Build history of the part. All positions in model axes, mm. Round coordinates to 2 decimals unless told otherwise and drop trailing zeros. Loops run counter-clockwise (first coordinate to the right, second up) from the corner with the lowest first, then second, coordinate; pieces in that order, holes last. Notation, with made-up numbers: (12.5, 33) - (49.5, 33) arc R18 cw to (49.5, 45) - close; hole circle Ø11 at (69.25, 8.5). An arc over 180 degrees is marked (long way). Put each result on its own line as item: value. Start each with the question number.
from build123d import *

# Parameters (mm, degrees)
BOSS_EXTRUDE1_DEPTH                             = 950
CBORE_FOR_M5_SOCKET_HEAD_CAP_SCREW2_D           = 5.5
CBORE_FOR_M5_SOCKET_HEAD_CAP_SCREW2_CBORE_D     = 10
CBORE_FOR_M5_SOCKET_HEAD_CAP_SCREW2_CBORE_DEPTH = 5
LPATTERN1_COUNT                                 = 16
LPATTERN1_PITCH                                 = 60


with BuildPart() as part:
    # Sketch1 → Boss-Extrude1 (new body)
    with BuildSketch(Plane.XY):
        Polygon((0, -9.237604307), (8, -4.618802154), (8, 4.618802154), (0, 9.237604307), (-8, 4.618802154), (-8, -4.618802154), align=None)
    extrude(amount=BOSS_EXTRUDE1_DEPTH)

    # CBORE for M5 Socket Head Cap Screw2 (through all)
    with Locations(Plane(origin=(8, 0, 925), x_dir=(0, 1, 0), z_dir=(1, 0, 0))):
        with Locations((0, 0)):
            cbore_for_m5_socket_head_cap_screw2 = CounterBoreHole(CBORE_FOR_M5_SOCKET_HEAD_CAP_SCREW2_D / 2, CBORE_FOR_M5_SOCKET_HEAD_CAP_SCREW2_CBORE_D / 2, CBORE_FOR_M5_SOCKET_HEAD_CAP_SCREW2_CBORE_DEPTH)

    # LPattern1: CBORE for M5 Socket Head Cap Screw2 ×16
    with Locations(*[(0, 0, -i * LPATTERN1_PITCH) for i in range(1, LPATTERN1_COUNT)]):
        add(cbore_for_m5_socket_head_cap_screw2, mode=Mode.SUBTRACT)


solid = part.part
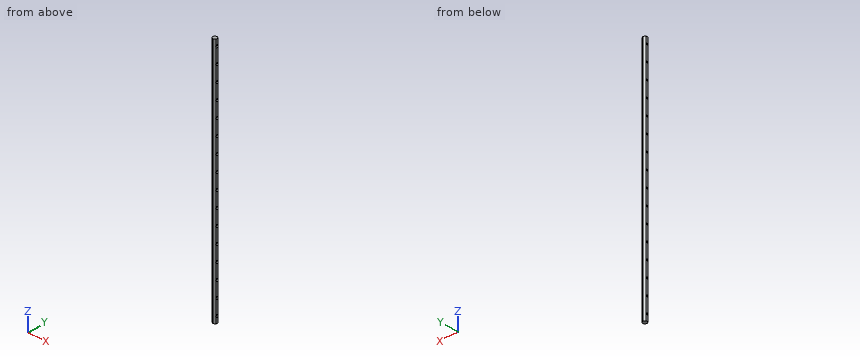
1) Slice it at A-A, the plane z = 541. Write the cut outline in (x, y), and give its area (3 significant figures).
2) Drill centre lines: line 1 (Y direction, x = -3, z = 625); line 2 (Y direction, x = 2.25, z = 209); line 3 (X direction, y = 6.25, z = 881). Where is each one in solid material? Low to high. Write a range as [from, to].
3) Drop flat-ended pins along their axis: pin 1 Ø9 at (y, z) = (0, 865) entering from +X; pin 2 Ø1 at (y, z) = (7, 113) entering from -X; pin 3 Ø1 at (y, z) = (6, 162.5) entering from +X; pin 4 Ø5 at (y, z) = (0, 205) entering from -X. Give the stop position or say it passes through.
Taken from the geometry:
1. outline: (-8, -4.62) - (0, -9.24) - (8, -4.62) - (8, 4.62) - (0, 9.24) - (-8, 4.62) - close
1. area: 222 mm2
2. line 1: y = [-7.51, -2.75], [2.75, 7.51]
2. line 2: y = [-7.94, 7.94]
2. line 3: x = [-5.17, 5.17]
3. pin 1: stops at x = 3
3. pin 2: stops at x = -4.74
3. pin 3: stops at x = 6.47
3. pin 4: passes through
